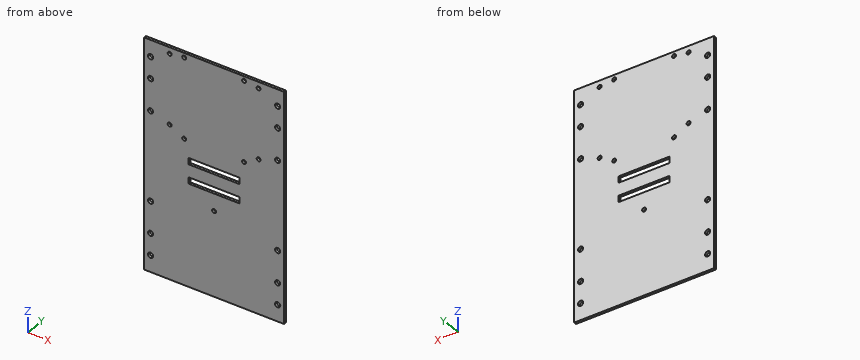
```python
from build123d import *

# Parameters (mm, degrees)
SKETCH1_W           = 55
SKETCH1_H           = 90.1
SKETCH1_R           = 2.05
BOSS_EXTRUDE2_DEPTH = 2
MIRROR1_OUTLINE_W   = 55
MIRROR1_OUTLINE_H   = 90.1
MIRROR1_OUTLINE_R   = 2.05
MIRROR1_DEPTH       = 2
SKETCH2_W           = 40.1
SKETCH2_H           = 5
CUT_EXTRUDE1_DEPTH  = 10
SKETCH3_R           = 1.55
CUT_EXTRUDE2_DEPTH  = 10


# Read off the part's stored shape, not the designer's step: Mirror1
with BuildPart() as part:
    # Sketch1 → Boss-Extrude2 (new body)
    with BuildSketch(Plane(origin=(0, 0, 0), x_dir=(1, 0, 0), z_dir=(0, 1, 0))):
        with Locations((27.5, 45.05)):
            Rectangle(SKETCH1_W, SKETCH1_H)
        with Locations(Location((50, 77.1, 0), (0, 0, 270))):
            Circle(SKETCH1_R, mode=Mode.SUBTRACT)
        with Locations(Location((50, 60.1, 0), (0, 0, 270))):
            Circle(SKETCH1_R, mode=Mode.SUBTRACT)
        with Locations(Location((50, 35, 0), (0, 0, 270))):
            Circle(SKETCH1_R, mode=Mode.SUBTRACT)
    extrude(amount=BOSS_EXTRUDE2_DEPTH)

    # Mirror1 outline → Mirror1 (add)
    with BuildSketch(Plane(origin=(0, 0, 0), x_dir=(1, 0, 0), z_dir=(0, 1, 0))):
        with Locations((-27.5, 45.05)):
            Rectangle(MIRROR1_OUTLINE_W, MIRROR1_OUTLINE_H)
        with Locations((-50, 35)):
            Circle(MIRROR1_OUTLINE_R, mode=Mode.SUBTRACT)
        with Locations((-50, 60.1)):
            Circle(MIRROR1_OUTLINE_R, mode=Mode.SUBTRACT)
        with Locations((-50, 77.1)):
            Circle(MIRROR1_OUTLINE_R, mode=Mode.SUBTRACT)
    extrude(amount=MIRROR1_DEPTH)

    # Mirror2: part across plane


with BuildPart() as part_1:
    add(part.part)
    add(part.part.mirror(Plane(origin=(0, 2, 0), x_dir=(1, 0, 0), z_dir=(0, 0, -1))))

    # Sketch2 → Cut-Extrude1 (cut)
    with BuildSketch(Plane(origin=(0, 2, 0), x_dir=(1, 0, 0), z_dir=(0, 1, 0))):
        with Locations((0, 7.5)):
            Rectangle(SKETCH2_W, SKETCH2_H)
        with Locations((0, -7.5)):
            Rectangle(SKETCH2_W, SKETCH2_H)
    extrude(amount=-CUT_EXTRUDE1_DEPTH, mode=Mode.SUBTRACT)

    # Sketch3 → Cut-Extrude2 (cut)
    with BuildSketch(Plane(origin=(0, 2, 0), x_dir=(1, 0, 0), z_dir=(0, 1, 0))):
        with Locations(Location((-35, -30.1, 0), (0, 0, 270))):
            Circle(SKETCH3_R)
        with Locations(Location((-35, -85.1, 0), (0, 0, 270))):
            Circle(SKETCH3_R)
        with Locations(Location((35, -30.1, 0), (0, 0, 270))):
            Circle(SKETCH3_R)
        with Locations(Location((35, -85.1, 0), (0, 0, 270))):
            Circle(SKETCH3_R)
        with Locations(Location((0, 23.55, 0), (0, 0, 270))):
            Circle(SKETCH3_R)
        with Locations(Location((23.55, -23.55, 0), (0, 0, 270))):
            Circle(SKETCH3_R)
        with Locations(Location((-23.55, -86.6, 0), (0, 0, 270))):
            Circle(SKETCH3_R)
        with Locations(Location((23.55, -86.6, 0), (0, 0, 270))):
            Circle(SKETCH3_R)
        with Locations(Location((-23.55, -23.55, 0), (0, 0, 270))):
            Circle(SKETCH3_R)
    extrude(amount=-CUT_EXTRUDE2_DEPTH, mode=Mode.SUBTRACT)


solid = part_1.part
```
Source: CAD feature listing. Evaluate the final solid. Frame: model axes, mm. Round coordinates to 2 decimals unless told otherwise and drop trailing zeros. Loops run counter-clockwise (first coordinate to the right, second up) from the corner with the lowest first, then second, coordinate; pieces in that order, holes last. Notation, with made-up numbers: M -30,-22 L 10,-22 A8 ccw 10,-8 Z; hole C -19,-35.5 d2. An arc over 180 degrees is marked long. Use a Markdown table: item, result. Add a question column.
1. Section query A-A on x = 50. Return the cut outline in (y, z).
2. Line query: line 1 (X direction, y = 0.8, z = 30.1); line 2 (Z direction, x = -17, y = 0.4); line 3 (X direction, y = 1.5, z = 77.1). Output: solid intervals per line, ascending.
3. Section query C-C on z = -35. Return the cut outline in (x, y).
4. Section query B-B on x = -14.5. Return the cut outline in (y, z), then the cut area to 3 significant figures.
5. Section query D-D on y = 0.6. Give the number of separate pieces and of enclosed holes in the cut face, then the cut area to 3 significant figures.
Reported:
| question | item | result |
|---|---|---|
| 1 | outline | M 0,-90.1 L 2,-90.1 L 2,-79.15 L 0,-79.15 Z; M 0,-75.05 L 2,-75.05 L 2,-62.15 L 0,-62.15 Z; M 0,-58.05 L 2,-58.05 L 2,-37.05 L 0,-37.05 Z; M 0,-32.95 L 2,-32.95 L 2,32.95 L 0,32.95 Z; M 0,37.05 L 2,37.05 L 2,58.05 L 0,58.05 Z; M 0,62.15 L 2,62.15 L 2,75.05 L 0,75.05 Z; M 0,79.15 L 2,79.15 L 2,90.1 L 0,90.1 Z |
| 2 | line 1 | x = -55 to -36.55, -33.45 to 33.45, 36.55 to 55 |
| 2 | line 2 | z = -90.1 to -10, -5 to 5, 10 to 90.1 |
| 2 | line 3 | x = -55 to -52.05, -47.95 to 47.95, 52.05 to 55 |
| 3 | outline | M -55,0 L -52.05,0 L -52.05,2 L -55,2 Z; M -47.95,0 L 47.95,0 L 47.95,2 L -47.95,2 Z; M 52.05,0 L 55,0 L 55,2 L 52.05,2 Z |
| 4 | outline | M 0,-90.1 L 2,-90.1 L 2,-10 L 0,-10 Z; M 0,-5 L 2,-5 L 2,5 L 0,5 Z; M 0,10 L 2,10 L 2,90.1 L 0,90.1 Z |
| 4 | area | 340 mm² |
| 5 | separate pieces | 1 |
| 5 | enclosed holes | 23 |
| 5 | area | 19,200 mm² |
